Geometry check sheet. Reference: the model listing, model coordinates, mm. A direction names the side the tool comes from. Give positions to 0.01 mm unless a question says otherwise; leave off trailing zeros. Write each loop counter-clockwise with the first axis right and the second up, starting at its lowest first coordinate (ties: lowest second). Pieces come first, ordered by that corner, then holes. Notation, with made-up numbers: (26, -28) -> (32, -28) arc R33 ccw to (32, 9) -> close; hole circle Ø4 at (-38.75, 62.25). An arc over 180 degrees is marked (long way). One line per item, written item: value.
from build123d import *

# Parameters (mm, degrees)
SKETCH1_W                                      = 150
SKETCH1_H                                      = 100
BOSS_EXTRUDE1_DEPTH                            = 8
CBORE_FOR_2_SOCKET_HEAD_CAP_SCREW1_D           = 2.4384
CBORE_FOR_2_SOCKET_HEAD_CAP_SCREW1_CBORE_D     = 4.7625
CBORE_FOR_2_SOCKET_HEAD_CAP_SCREW1_CBORE_DEPTH = 2.1844
F_2_56_TAPPED_HOLE1_D                          = 1.778
F_2_56_TAPPED_HOLE1_DEPTH                      = 20
F_2_56_TAPPED_HOLE1_TIP                        = 0.53416509
SKETCH7_R                                      = 6.5
SKETCH7_R_2                                    = 3.25
BNC_PIEZO_BNC_THRU_HOLES_DEPTH                 = 9
F_4_40_TAPPED_HOLE1_D                          = 2.2606
F_4_40_TAPPED_HOLE1_CSINK_D                    = 4.1148
F_4_40_TAPPED_HOLE1_CSINK_ANGLE                = 90
SKETCH7_3_R                                    = 6.5
SKETCH7_3_R_2                                  = 3.25
CUT_EXTRUDE2_DEPTH                             = 5


with BuildPart() as part:
    # Sketch1 → Boss-Extrude1 (new body)
    with BuildSketch(Plane.XY):
        with Locations((75, 50)):
            Rectangle(SKETCH1_W, SKETCH1_H)
    extrude(amount=BOSS_EXTRUDE1_DEPTH)

    # CBORE for #2 Socket Head Cap Screw1 (through all)
    with Locations(Plane(origin=(0, 0, 0), x_dir=(-1, 0, 0), z_dir=(0, 0, -1))):
        with Locations((-132, 4), (-18, 4), (-4, 90), (-146, 90), (-146, 10), (-4, 10), (-75, 4)):
            CounterBoreHole(CBORE_FOR_2_SOCKET_HEAD_CAP_SCREW1_D / 2, CBORE_FOR_2_SOCKET_HEAD_CAP_SCREW1_CBORE_D / 2, CBORE_FOR_2_SOCKET_HEAD_CAP_SCREW1_CBORE_DEPTH)

    # #2-56 Tapped Hole1
    with Locations(Plane(origin=(0, 100, 0), x_dir=(1, 0, 0), z_dir=(0, 1, 0))):
        with Locations((18, -4), (75, -4), (132, -4)):
            Hole(F_2_56_TAPPED_HOLE1_D / 2, depth=F_2_56_TAPPED_HOLE1_DEPTH)
            with Locations((0, 0, -(F_2_56_TAPPED_HOLE1_DEPTH + F_2_56_TAPPED_HOLE1_TIP / 2))):  # 118° drill point
                Cone(0, F_2_56_TAPPED_HOLE1_D / 2, F_2_56_TAPPED_HOLE1_TIP, mode=Mode.SUBTRACT)

    # Sketch7 → BNC & piezo & BNC thru holes (cut, through all)
    with BuildSketch(Plane.XY.offset(8)):
        with BuildLine():
            Line((45.313838353, 68.75), (52.313838353, 68.75))
            ThreePointArc((52.313838353, 68.75), (53.728051916, 68.164213562), (54.313838353, 66.75))
            Line((54.313838353, 66.75), (54.313838353, 51.25))
            ThreePointArc((54.313838353, 51.25), (53.728051916, 49.835786438), (52.313838353, 49.25))
            Line((52.313838353, 49.25), (45.313838353, 49.25))
            ThreePointArc((45.313838353, 49.25), (43.899624791, 49.835786438), (43.313838353, 51.25))
            Line((43.313838353, 51.25), (43.313838353, 66.75))
            ThreePointArc((43.313838353, 66.75), (43.899624791, 68.164213562), (45.313838353, 68.75))
        make_face()
        with BuildLine():
            Line((65.313838353, 68.75), (72.313838353, 68.75))
            ThreePointArc((72.313838353, 68.75), (73.728051916, 68.164213562), (74.313838353, 66.75))
            Line((74.313838353, 66.75), (74.313838353, 51.25))
            ThreePointArc((74.313838353, 51.25), (73.728051916, 49.835786438), (72.313838353, 49.25))
            Line((72.313838353, 49.25), (65.313838353, 49.25))
            ThreePointArc((65.313838353, 49.25), (63.899624791, 49.835786438), (63.313838353, 51.25))
            Line((63.313838353, 51.25), (63.313838353, 66.75))
            ThreePointArc((63.313838353, 66.75), (63.899624791, 68.164213562), (65.313838353, 68.75))
        make_face()
        with Locations((93.813838353, 59)):
            Circle(SKETCH7_R)
        with Locations((113.313838353, 59)):
            Circle(SKETCH7_R)
        with Locations((48.813838353, 27.1)):
            Circle(SKETCH7_R_2)
    extrude(amount=-BNC_PIEZO_BNC_THRU_HOLES_DEPTH, mode=Mode.SUBTRACT)

    # #4-40 Tapped Hole1 (through all)
    with Locations(Plane.XY.offset(8)):
        with Locations((48.813838353, 71.5), (68.813838353, 71.5), (68.813838353, 46.5), (48.813838353, 46.5)):
            CounterSinkHole(F_4_40_TAPPED_HOLE1_D / 2, F_4_40_TAPPED_HOLE1_CSINK_D / 2, counter_sink_angle=F_4_40_TAPPED_HOLE1_CSINK_ANGLE)

    # Sketch7<3> → Cut-Extrude2 (cut)
    with BuildSketch(Plane.XY.offset(8)):
        with BuildLine():
            Line((38.813838353, 85.1), (123.313838353, 85.1))
            ThreePointArc((123.313838353, 85.1), (126.849372259, 83.635533906), (128.313838353, 80.1))
            Line((128.313838353, 80.1), (128.313838353, 17.8))
            ThreePointArc((128.313838353, 17.8), (126.849372259, 14.264466094), (123.313838353, 12.8))
            Line((123.313838353, 12.8), (38.813838353, 12.8))
            ThreePointArc((38.813838353, 12.8), (35.278304447, 14.264466094), (33.813838353, 17.8))
            Line((33.813838353, 17.8), (33.813838353, 80.1))
            ThreePointArc((33.813838353, 80.1), (35.278304447, 83.635533906), (38.813838353, 85.1))
        make_face()
        with Locations((93.813838353, 59)):
            Circle(SKETCH7_3_R, mode=Mode.SUBTRACT)
        with Locations((113.313838353, 59)):
            Circle(SKETCH7_3_R, mode=Mode.SUBTRACT)
        with Locations((48.813838353, 27.1)):
            Circle(SKETCH7_3_R_2, mode=Mode.SUBTRACT)
        with BuildLine():
            Line((45.313838353, 68.75), (52.313838353, 68.75))
            ThreePointArc((52.313838353, 68.75), (53.728051916, 68.164213562), (54.313838353, 66.75))
            Line((54.313838353, 66.75), (54.313838353, 51.25))
            ThreePointArc((54.313838353, 51.25), (53.728051916, 49.835786438), (52.313838353, 49.25))
            Line((52.313838353, 49.25), (45.313838353, 49.25))
            ThreePointArc((45.313838353, 49.25), (43.899624791, 49.835786438), (43.313838353, 51.25))
            Line((43.313838353, 51.25), (43.313838353, 66.75))
            ThreePointArc((43.313838353, 66.75), (43.899624791, 68.164213562), (45.313838353, 68.75))
        make_face(mode=Mode.SUBTRACT)
        with BuildLine():
            Line((65.313838353, 68.75), (72.313838353, 68.75))
            ThreePointArc((72.313838353, 68.75), (73.728051916, 68.164213562), (74.313838353, 66.75))
            Line((74.313838353, 66.75), (74.313838353, 51.25))
            ThreePointArc((74.313838353, 51.25), (73.728051916, 49.835786438), (72.313838353, 49.25))
            Line((72.313838353, 49.25), (65.313838353, 49.25))
            ThreePointArc((65.313838353, 49.25), (63.899624791, 49.835786438), (63.313838353, 51.25))
            Line((63.313838353, 51.25), (63.313838353, 66.75))
            ThreePointArc((63.313838353, 66.75), (63.899624791, 68.164213562), (65.313838353, 68.75))
        make_face(mode=Mode.SUBTRACT)
    extrude(amount=-CUT_EXTRUDE2_DEPTH, mode=Mode.SUBTRACT)


solid = part.part
1) Sectioned sample at B-B on y = 22. Record the cut outline in (x, z), plus the area to 4 significant figures.
Verdict:
outline: (0, 0) -> (150, 0) -> (150, 8) -> (128.31, 8) -> (128.31, 3) -> (33.81, 3) -> (33.81, 8) -> (0, 8) -> close
area: 727.5 mm^2
2) Sectioned sample at C-C on x = 90.5. Record the cut outline in (y, z).
Verdict:
outline: (0, 0) -> (53.41, 0) -> (53.41, 3) -> (12.8, 3) -> (12.8, 8) -> (0, 8) -> close; (64.59, 0) -> (100, 0) -> (100, 8) -> (85.1, 8) -> (85.1, 3) -> (64.59, 3) -> close
3) Tool access check on faces 1 (the flat face through (24, 51, 8)), 2 (the flat face through (74, 0, 4)), 3 (the flat face through (33.814, 49, 6)), 4 (the cylindrical face through (18.31, 6.36, 1.08)), 5 (the flat face through (54.314, 59, 2)). Record the directions out of +Z, -Z, +X, -X, +Y, -Y that give a thin tool (end or side, any length) a straight path to the whole face; none if there is none.
Verdict:
face 1: +Z, +X, -X, +Y, -Y
face 2: +Z, -Z, +X, -X, -Y
face 3: +Z
face 4: -Z
face 5: +Z, -Z
4) Depth check by flat-ended pin: pin 1 Ø1.4 at (x, y) = (133, 3.5) entering from -Z; pin 2 Ø10 at (x, y) = (39.5, 66.5) entering from +Z. Enter the tip coordinate at first touch or a pass-through.
Verdict:
pin 1: z = 2.18
pin 2: z = 3
5) Sectioned sample at A-A on z = 6.25. Give the number of separate pieces and of enclosed holes in the cut face, plus the area to 3 significant figures.
Verdict:
separate pieces: 1
enclosed holes: 8
area: 8,160 mm^2
6) Scan lines: probe 1 along X at (y, z) = (90, 3.9); probe 2 along X at (y, z) = (90, 5.7); probe 3 along X at (y, z) = (94, 4). Record each from-to range of solid material in increasing order.
Verdict:
probe 1: 0 to 2.78, 5.22 to 17.12, 18.88 to 74.12, 75.88 to 131.12, 132.88 to 144.78, 147.22 to 150
probe 2: 0 to 2.78, 5.22 to 144.78, 147.22 to 150
probe 3: 0 to 17.11, 18.89 to 74.11, 75.89 to 131.11, 132.89 to 150
